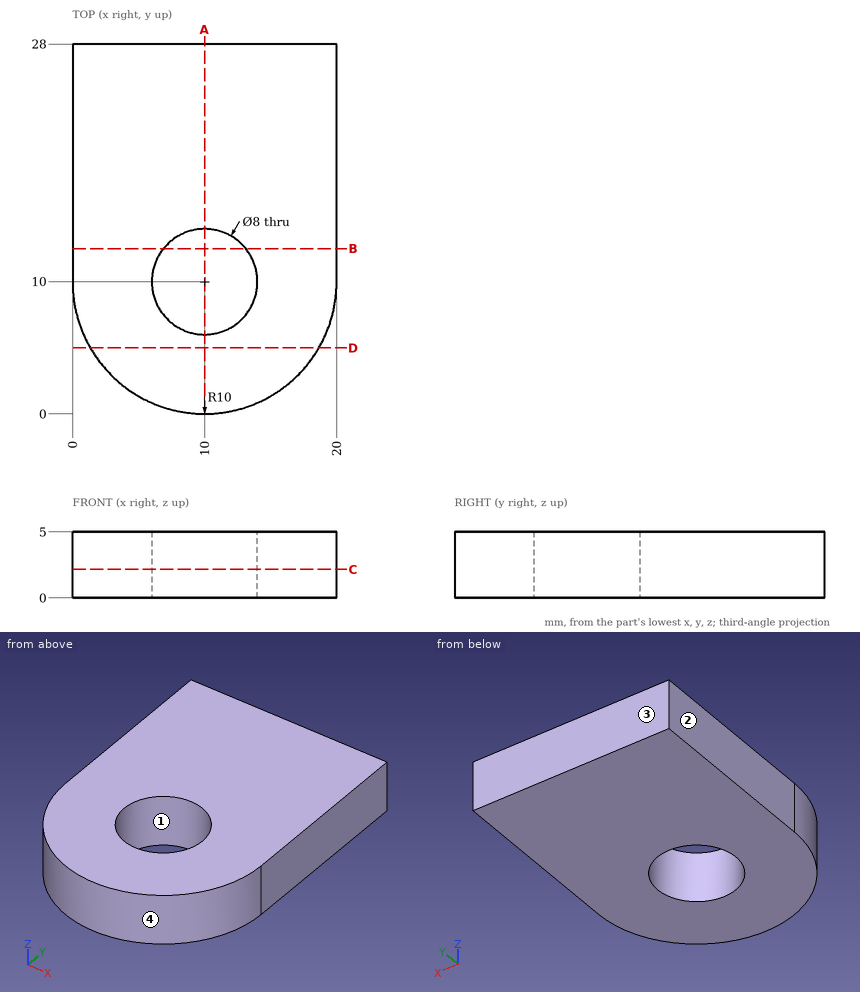
Verification items for this drawing (mm, ordinates from the low corner). Coordinates: 2 decimals unless noted, no trailing zeros. Order: outer loops, then holes, each group sorted by start corner. A loop starts at its lowest first (then second) coordinate and runs counter-clockwise, first axis right, second up. Notation, with made-up numbers: (38, 76.5) -> (86, 76.5) arc R11 ccw to (86, 95.5) -> close; hole circle Ø6 at (-1.5, -19.5). An arc over 180 degrees is marked (long way). Put each result on its own line as item: value. Start each with the question number.
1. Cross-section at A-A, the plane x = 10. Record the boundary of the cut face in (y, z), then the cut area to 3 significant figures.
2. Material ranges on L1, parallel to Y at x = 10, z = 3.9; L2, parallel to Y at x = 6.5, z = 2.45; L3, parallel to X at y = 8, z = 4.1, recorded low to high. Write a range as [from, to].
3. Cross-section at B-B, the plane y = 12.5. Record the boundary of the cut face in (x, z), then the cut area to 3 significant figures.
4. Cross-section at D-D, the plane y = 5. Record the boundary of the cut face in (x, z), then the cut area to 3 significant figures.
5. Cross-section at C-C, the plane z = 2.15. Record the boundary of the cut face in (x, y).
6. Mould release check, pull along Y, two halves, no side actions. Record for the marked faces 1, 2, 3 and 4: released by +Y, released by -Y, zero draft, split by the parting line, or undercut.
Computed:
1. outline: (0, 0) -> (6, 0) -> (6, 5) -> (0, 5) -> close; (14, 0) -> (28, 0) -> (28, 5) -> (14, 5) -> close
1. area: 100 mm2
2. L1: [0, 6], [14, 28]
2. L2: [0.63, 8.06], [11.94, 28]
2. L3: [0.2, 6.54], [13.46, 19.8]
3. outline: (0, 0) -> (6.88, 0) -> (6.88, 5) -> (0, 5) -> close; (13.12, 0) -> (20, 0) -> (20, 5) -> (13.12, 5) -> close
3. area: 68.8 mm2
4. outline: (1.34, 0) -> (18.66, 0) -> (18.66, 5) -> (1.34, 5) -> close
4. area: 86.6 mm2
5. outline: (0, 10) arc R10 ccw to (20, 10) -> (20, 28) -> (0, 28) -> close; hole circle Ø8 at (10, 10)
6. face 1: undercut
6. face 2: zero draft
6. face 3: released by +Y
6. face 4: released by -Y
